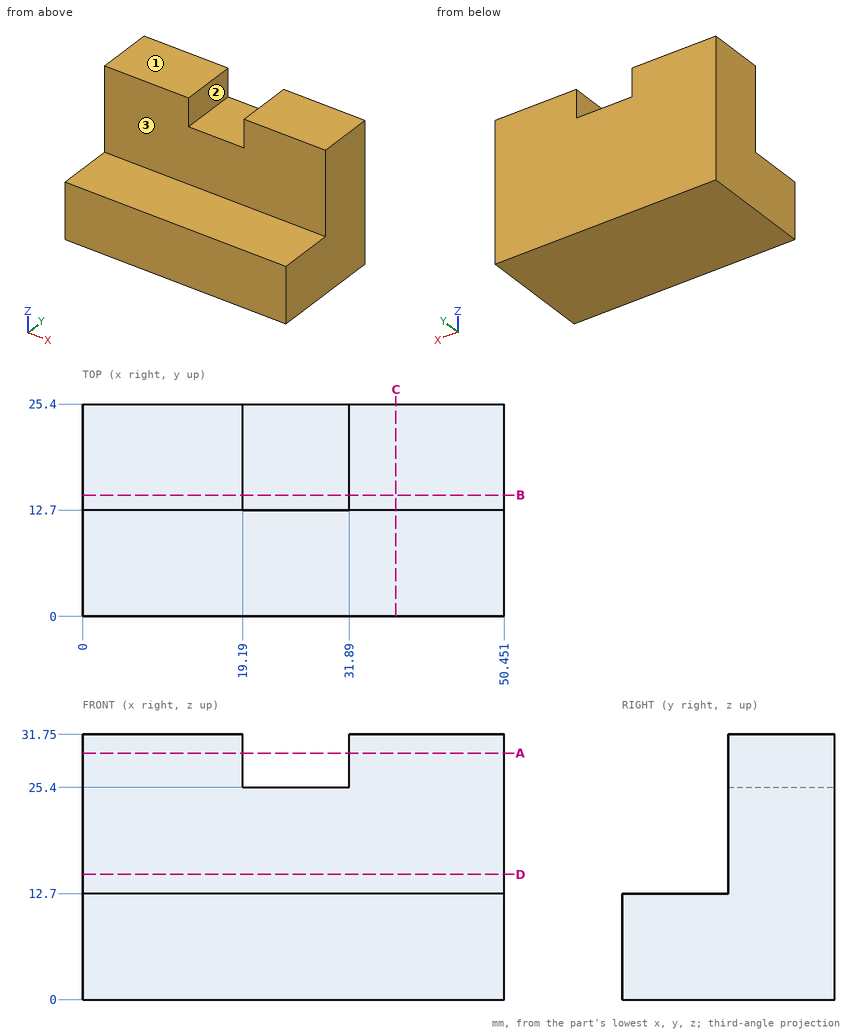
Job drawing, mm, ordinate dimensions from the low corner. One solid piece. A direction names the side the tool comes from. Round coordinates to 2 decimals unless told otherwise and drop trailing zeros. Order: outer loops, then holes, each group sorted by start corner. A loop starts at its lowest first (then second) coordinate and runs counter-clockwise, first axis right, second up. Notation, with made-up numbers: (-8.5, 63.5) -> (14.5, 63.5) arc R22 ccw to (14.5, 74.5) -> close; hole circle Ø9 at (28.5, -17). An arc over 180 degrees is marked (long way). Write item = value, one per line.
(1) Cut at A-A (z = 29.5). Write the cut outline in (x, y), plus the area to 3 significant figures.
Answers follow:
outline = (0, 12.7) -> (19.19, 12.7) -> (19.19, 25.4) -> (0, 25.4) -> close; (31.89, 12.7) -> (50.45, 12.7) -> (50.45, 25.4) -> (31.89, 25.4) -> close
area = 479 mm²
(2) Cut at B-B (y = 14.5). Write the cut outline in (x, z), plus the area to 3 significant figures.
Answers follow:
outline = (0, 0) -> (50.45, 0) -> (50.45, 31.75) -> (31.89, 31.75) -> (31.89, 25.4) -> (19.19, 25.4) -> (19.19, 31.75) -> (0, 31.75) -> close
area = 1,520 mm²
(3) Flat gauge pins, fed straight in: P1, Ø1, axis at x = 27.5, z = 23, coming from the -Y side; P2, Ø6.5, axis at x = 26, y = 18, coming from the +Z side; P3, Ø6.5, axis at x = 21, y = 6, coming from the +Z side. Where does each tip first touch, or does it go through?
Answers follow:
P1 = 12.7
P2 = 25.4
P3 = 12.7
(4) Cut at D-D (z = 15). Write the cut outline in (x, y), plus the area to 3 significant figures.
Answers follow:
outline = (0, 12.7) -> (50.45, 12.7) -> (50.45, 25.4) -> (0, 25.4) -> close
area = 641 mm²
(5) Cut at C-C (x = 37.5). Write the cut outline in (y, z).
Answers follow:
outline = (0, 0) -> (25.4, 0) -> (25.4, 31.75) -> (12.7, 31.75) -> (12.7, 12.7) -> (0, 12.7) -> close
(6) 3-axis set-ups, long thin cutter, end or side, ignore diameter. For the marked faces 1, 2 and 3: which of +Z, -Z, +X, -X, +Y, -Y reach the whole face in a straight line?
Answers follow:
face_1 = +Z, +X, -X, +Y, -Y
face_2 = +Z, +Y, -Y
face_3 = +Z, +X, -X, -Y
(7) Drill centre lines: L1, parallel to Z at x = 24, y = 21.75; L2, parallel to Y at x = 28, z = 18; L3, parallel to Z at x = 27.5, y = 7.5. Where is each one in solid material? Low to high.
Answers follow:
L1 = 0 to 25.4
L2 = 12.7 to 25.4
L3 = 0 to 12.7
